```python
from build123d import *

# Parameters (mm, degrees)
BOSS_EXTRUDE1_DEPTH = 6
SKETCH3_R           = 4.55625
CUT_EXTRUDE1_DEPTH  = 99


with BuildPart() as part:
    # Sketch1 → Revolve1 (revolve)
    with BuildSketch(Plane.XY, mode=Mode.PRIVATE) as revolve1_sk:
        Polygon((0, 13), (5.55625, 13), (5.55625, 0), (10, 0), (10, -28), (5.55625, -38), (5.55625, -88), (0, -88), align=None)
    revolve(revolve1_sk.sketch.rotate(Axis((0, 13, 0), (0, -1, 0)), 180), axis=Axis((0, 13, 0), (0, -1, 0)))

    # Sketch2 → Boss-Extrude1 (add)
    with BuildSketch(Plane(origin=(0, 0, 0), x_dir=(1, 0, 0), z_dir=(0, 1, 0))):
        Polygon((12.701705922, 0), (6.350852961, 11), (-6.350852961, 11), (-12.701705922, 0), (-6.350852961, -11), (6.350852961, -11), align=None)
    extrude(amount=-BOSS_EXTRUDE1_DEPTH)

    # Sketch3 → Cut-Extrude1 (cut)
    with BuildSketch(Plane(origin=(0, 13, 0), x_dir=(1, 0, 0), z_dir=(0, 1, 0))):
        with Locations(Location((0, 0, 0), (0, 0, 180))):
            Circle(SKETCH3_R)
    extrude(amount=-CUT_EXTRUDE1_DEPTH, mode=Mode.SUBTRACT)


solid = part.part
```
The listing builds one solid part. Answer for the finished solid, in the listing's coordinates (mm). A direction names the side the tool comes from. Give positions to 0.01 mm unless a question says otherwise; leave off trailing zeros. Order: outer loops, then holes, each group sorted by start corner. A loop starts at its lowest first (then second) coordinate and runs counter-clockwise, first axis right, second up. Notation, with made-up numbers: (4, -33) - (49, -33) arc R24 cw to (49, -3) - close; hole circle Ø5 at (-18, 11). An arc over 180 degrees is marked (long way). Answer in a Markdown table with one row per item. Add a question column.
Q1. The part is cut by section A-A (x = 0). Determine the outline of the cut face in (y, z).
Q2. Given P1, Ø2, axis at x = 5.5, y = -13.5, coming from the +Z side; P2, Ø4.5, axis at x = 0, z = 1.5, coming from the +Y side; P3, Ø5, axis at x = 5, z = 6.5, coming from the -Y side, each flat-ended and moving along its own axis, determine where each tip first touches the part or whether it passes through.
Q3. For a pull along Z with two mould halves and no side action, classify faces 4 (the flat face through (0, 13, -5)), 5 (the cylindrical face through (-2.102, -35.807, -4.042)), 6 (the flat face through (-9.571, -2.958, 5.423)), 7 (the cylindrical face through (4.095, -63.35, -3.755)) as released by +Z, released by -Z, zero draft, split by the parting line, or undercut.
Q4. The part is cut by section C-C (y = -30.5). Determine the outline of the cut face in (x, z), then the cut area to 3 significant figures.
Q5. The part is cut by section B-B (y = -62). Determine the outline of the cut face in (x, z).
Q6. Find the intervals of material crossed by line 1 along Z through (x, y) = (0, -17.5); line 2 along Z through (x, y) = (0, -62.5); line 3 along Y through (x, z) = (3, 3), in increasing order. Write a range as [from, to].
Q7. Which of the six approach directions +Z, -Z, +X, -X, +Y, -Y give full straight-line access (tool end or side, diameter ignored) to faces 1 (the flat face through (-9.48, -2.96, -5.58)), 2 (the cylindrical face through (4.095, 6.409, -3.755)), 3 (the flat face through (8.4, -6, -5.8))?
Determined:
| question | item | result |
|---|---|---|
| 1 | outline | (-88, -5.56) - (-38, -5.56) - (-28, -10) - (-6, -10) - (-6, -11) - (0, -11) - (0, -5.56) - (13, -5.56) - (13, -4.56) - (-86, -4.56) - (-86, 4.56) - (13, 4.56) - (13, 5.56) - (0, 5.56) - (0, 11) - (-6, 11) - (-6, 10) - (-28, 10) - (-38, 5.56) - (-88, 5.56) - close |
| 2 | P1 | stops at z = 8.93 |
| 2 | P2 | stops at y = -86 |
| 2 | P3 | stops at y = -37.68 |
| 3 | face 4 | zero draft |
| 3 | face 5 | undercut |
| 3 | face 6 | released by +Z |
| 3 | face 7 | split by the parting line |
| 4 | outline | circle Ø17.78 at (0, 0); hole circle Ø9.11 at (0, 0) |
| 4 | area | 183 mm² |
| 5 | outline | circle Ø11.11 at (0, 0); hole circle Ø9.11 at (0, 0) |
| 6 | line 1 | z = [-10, -4.56], [4.56, 10] |
| 6 | line 2 | z = [-5.56, -4.56], [4.56, 5.56] |
| 6 | line 3 | y = [-88, -86] |
| 7 | face 1 | -Z, -X, +Y, -Y |
| 7 | face 2 | +Y |
| 7 | face 3 | -Y |
